```python
from build123d import *

# Parameters (mm, degrees)
SKETCH001_W     = 178.4
SKETCH001_H     = 120.07
SKETCH001_W_2   = 164.7
SKETCH001_H_2   = 98.22
PAD_DEPTH       = 2
SKETCH_W        = 178.4
SKETCH_H        = 120.07
PAD001_DEPTH    = 1.6
SKETCH009_W     = 5
SKETCH009_H     = 4
POCKET_DEPTH    = 2.9
SKETCH010_W     = 2.5
SKETCH010_H     = 1.8
POCKET001_DEPTH = 5
SKETCH011_R     = 1
PAD009_DEPTH    = 1.5


with BuildPart() as part:
    # Sketch001 (on Face45 of Binder) → Pad (new body)
    with BuildSketch(Plane.XY.offset(1.19)):
        with Locations((0, -0.305)):
            Rectangle(SKETCH001_W, SKETCH001_H)
        with Locations((0, 3.77)):
            Rectangle(SKETCH001_W_2, SKETCH001_H_2, mode=Mode.SUBTRACT)
    extrude(amount=PAD_DEPTH)

    # Sketch (on Face9 of Pad) → Pad001 (join)
    with BuildSketch(Plane(origin=(0, 0, 1.19), x_dir=(1, 0, 0), z_dir=(0, 0, -1))):
        with Locations((0, 0.305)):
            Rectangle(SKETCH_W, SKETCH_H)
        Polygon((-85.35, 55.86), (-85.35, -55.86), (85.35, -55.86), (85.35, 55.86), (11.4649, 55.86), (11.4649, 59.34), (-11.4649, 59.34), (-11.4649, 55.86), align=None, mode=Mode.SUBTRACT)
    extrude(amount=PAD001_DEPTH)

    # Sketch009 (on Face1 of Pad001) → Pocket (cut)
    with BuildSketch(Plane(origin=(0, 0, -0.41), x_dir=(1, 0, 0), z_dir=(0, 0, -1))):
        with Locations((85.7, -56.73)):
            Rectangle(SKETCH009_W, SKETCH009_H)
    extrude(amount=-POCKET_DEPTH, mode=Mode.SUBTRACT)

    # Sketch010 (on Face19 of Pocket) → Pocket001 (cut)
    with BuildSketch(Plane(origin=(0, 0, 1.19), x_dir=(1, 0, 0), z_dir=(0, 0, -1))):
        with Locations((86.14, -57.44)):
            Rectangle(SKETCH010_W, SKETCH010_H)
    extrude(amount=-POCKET001_DEPTH, mode=Mode.SUBTRACT)

    # Sketch011 (on Face1 of Pocket001) → Pad009 (join)
    with BuildSketch(Plane(origin=(0, 0, -0.41), x_dir=(1, 0, 0), z_dir=(0, 0, -1))):
        with Locations((-29.2, 57.84)):
            Circle(SKETCH011_R)
        with Locations((29.2, 57.84)):
            Circle(SKETCH011_R)
        with Locations((-29.2, -57.23)):
            Circle(SKETCH011_R)
        with Locations((29.2, -57.23)):
            Circle(SKETCH011_R)
        with Locations((-86.7, -24.73)):
            Circle(SKETCH011_R)
        with Locations((-86.7, 25.34)):
            Circle(SKETCH011_R)
        with Locations((86.7, 25.34)):
            Circle(SKETCH011_R)
        with Locations((86.7, -24.73)):
            Circle(SKETCH011_R)
    extrude(amount=PAD009_DEPTH)


solid = part.part
```
Can you work these out from the model? Positions are in its coordinate system, mm. A direction names the side the tool comes from. Give positions to 0.01 mm unless a question says otherwise; leave off trailing zeros. Loops run counter-clockwise (first coordinate to the right, second up) from the corner with the lowest first, then second, coordinate; pieces in that order, holes last. Notation, with made-up numbers: M 48.25,81 L 95.25,81 A18 cw 95.25,88 Z; hole C 33.25,49.5 d4. An arc over 180 degrees is marked long. One line per question, with ' | ' between items. Start each with the question number.
Q1. If we section it at A-A (x = 48): Please give me the cut outline in (y, z), plus the area to 3 significant figures.
Q2. If we mould it in two halves opening along Y, with no side actions, what happens to faces 3 (the flat face through (86, 56, 2.49)), 4 (the flat face through (-89.2, 1, 1)), 5 (the flat face through (-1, 59.73, 1)), 6 (the flat face through (-1, -60.34, 1))? For each: +Y half, -Y half, draft (parallel to the pull), parting line (faces both ways), or undercut.
Q3. For pin 1 Ø1.2 at (x, y) = (85.5, 57) entering from -Z, with a flat end and sliding along its axis, tell me the tip position at first contact or that it passes through.
Q4. If I drill on line 1 (X direction, y = -4, z = 1.45); line 2 (X direction, y = -30, z = 0.8); line 3 (Y direction, x = 23, z = 0.95), over which ranges is the centre line in solid material (lowest first)? Write a range as from..to.
Q5. For faces 1 (the flat face through (89.2, 1, 1)), 2 (the flat face through (0, 57, -0.41)), which set-ups out of +Z, -Z, +X, -X, +Y, -Y let a thin tool reach every point of the face, with its end or its side?
Q6. If we section it at B-B (y = -37): Please give me the cut outline in (x, z).
Computed:
1) outline: M -60.34,-0.41 L -55.86,-0.41 L -55.86,1.19 L -45.34,1.19 L -45.34,3.19 L -60.34,3.19 Z; M 52.88,1.19 L 55.86,1.19 L 55.86,-0.41 L 59.73,-0.41 L 59.73,3.19 L 52.88,3.19 Z | area: 57.1 mm²
2) face 3: undercut | face 4: draft | face 5: +Y half | face 6: -Y half
3) pin 1: stops at z = 2.49
4) line 1: x = -89.2..-82.35, 82.35..89.2 | line 2: x = -89.2..-85.35, 85.35..89.2 | line 3: y = -60.34..-55.86, 55.86..59.73
5) face 1: +Z, -Z, +X, +Y, -Y | face 2: -Z
6) outline: M -89.2,-0.41 L -85.35,-0.41 L -85.35,1.19 L -82.35,1.19 L -82.35,3.19 L -89.2,3.19 Z; M 82.35,1.19 L 85.35,1.19 L 85.35,-0.41 L 89.2,-0.41 L 89.2,3.19 L 82.35,3.19 Z
